Autodesk Inventor part; units mm, degrees
ref_plane "YZ Plane" through (0, 0, 0) normal (1, 0, 0) x (0, 1, 0)
ref_plane "XZ Plane" through (0, 0, 0) normal (0, 1, 0) x (-1, 0, 0)
ref_plane "XY Plane" through (0, 0, 0) normal (0, 0, 1) x (1, 0, 0)
sketch "Sketch1" plane through (0, 0, 0) normal (0, 0, 1) x (1, 0, 0)
  line L0 (0, 0) -> (60, 0)
  line L1 (0, 126.1861) -> (0, 150)
  line L2 (0, 18.2402) -> (0, 0)
  line L3 (0, 126.1861) -> (0, 18.2402)
  line L4 (70, 7.0021) -> (70, 100.5361)
  arc A0 (70, 100.5361) -> (0, 150) centre (14.4108, 96.1307) ccw
  arc A1 (60, 0) -> (70, 7.0021) centre (57.6261, 14.0321) ccw
  point P0 (84.7515, 38.5438)
  dimension "d1" = 60
  dimension "d2" = 150
  dimension "d22" = 10
revolve "Revolution1" add sketch "Sketch1" angle 360 about axis through (0, 126.1861, 0) along (0, -1, 0)
sketch "Sketch2" plane through (0, 0, 0) normal (1, 0, 0) x (0, 1, 0)
  line L0 (0, 75) -> (0, -75)
  circle A0 centre (75, 0) radius 60
  point P0 (0, 0)
  point P1 (150, 0)
  dimension "d4" = 120
  dimension "d25" = 75
extrude "Extrusion1" add sketch "Sketch2" along normal blind 72
hole "Hole1" at (72, 75, 0) direction (-1, 0, 0) diameter 108 depth 45
properties part number "tete"
Input: part model. Units: mm. Frame: model coordinates. A direction names the side the tool comes from. Round coordinates to 2 decimals unless told otherwise and drop trailing zeros. Loops run counter-clockwise (first coordinate to the right, second up) from the corner with the lowest first, then second, coordinate; pieces in that order, holes last. Notation, with made-up numbers: (-5.5, 0.25) -> (49.5, 0.25) arc R18 ccw to (49.5, 8.25) -> close; hole circle Ø3 at (-25, 43). An arc over 180 degrees is marked (long way). One line per item, written item: value.
(1) Section C-C (y = 52). Return the cut outline in (x, z), plus the area to 3 significant figures.
Geometry check:
outline: (27, -48.86) -> (27, 48.86) -> (72, 48.86) -> (72, 55.42) -> (42.77, 55.42) arc R70 ccw (long way) to (42.77, -55.42) -> (72, -55.42) -> (72, -48.86) -> close
area: 12,100 mm2
(2) Set-up query: faces 4 (the face through (49.185, 127.716, 11.706)), 5 (the face through (72, 21, 9)). Return all of +Z, -Z, +X, -X, +Y, -Y with unobstructed straight access to the full face (end or side cutting, diameter ignored); none if empty.
Geometry check:
face 4: +X
face 5: +Z, -Z, +X, +Y, -Y
(3) Mould query, pull axis Z, two halves, no side actions, for faces 1 (the face through (57.77, 132.23, -18.02)), 2 (the face through (-1, 0, 1)), 3 (the face through (27, 74, 1)). Classes: pulls with the +Z half, pulls with the -Z half, needs draft (parallel to the pull), parting line crosses it, or undercut.
Geometry check:
face 1: parting line crosses it
face 2: needs draft
face 3: undercut
(4) Section B-B (y = 10). Return the cut outline in (x, z), plus the area to 3 significant figures.
Geometry check:
outline: circle Ø140 at (0, 0)
area: 15,400 mm2
(5) Section A-A (y = 75). Return the cut outline in (x, z), plus the area to 3 significant figures.
Geometry check:
outline: (27, -54) -> (27, 54) -> (72, 54) -> (72, 60) -> (36.06, 60) arc R70 ccw (long way) to (36.06, -60) -> (72, -60) -> (72, -54) -> close
area: 12,000 mm2
(6) Material intervals for line 1 (Z direction, x = 61.5, y = 75); line 2 (Z direction, x = 44.5, y = 31); line 3 (Y direction, x = 52, z = 35), sorted ascending. Write a range as [from, to].
Geometry check:
line 1: [-60, -54], [54, 60]
line 2: [-54.03, -31.3], [31.3, 54.03]
line 3: [0.73, 33.88], [116.12, 124.05]
(7) Pin query (flat end, axial travel): pin 1 (12 mm diameter, centred on x = 40, z = -51, fed in from +Y); pin 2 (1.5 mm diameter, centred on x = 43.5, z = 35.5, fed in from +Y); pin 3 (12 mm diameter, centred on y = 89.5, z = 10, fed in from +X). Return the tip coordinate at first contact, or that it passes through.
Geometry check:
pin 1: y = 129.86
pin 2: y = 133.94
pin 3: x = 27
